Here's how the part is built. I have some questions about the finished solid (model axes, mm). Face numbers are marked on the shaded views. Round coordinates to 2 decimals unless told otherwise and drop trailing zeros. Loops run counter-clockwise (first coordinate to the right, second up) from the corner with the lowest first, then second, coordinate; pieces in that order, holes last. Notation, with made-up numbers: M 66.5,16 L 87.5,16 A16 cw 87.5,24 Z; hole C -15.75,-25 d9. An arc over 180 degrees is marked long. Use a Markdown table: item, result.
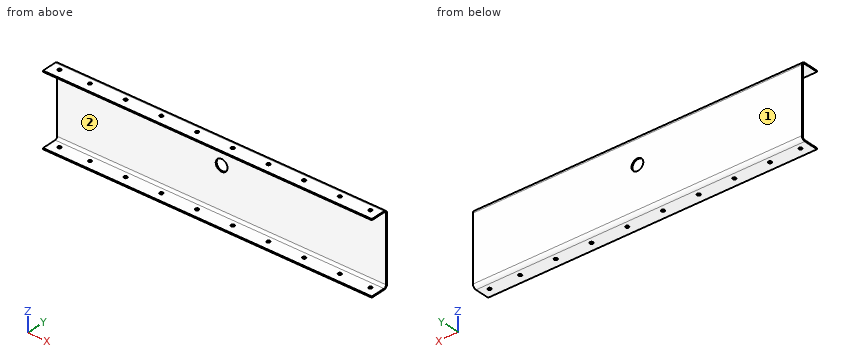
```python
from build123d import *

# Parameters (mm, degrees)
F1_DEPTH = 1400
F2_R     = 25
F3_DEPTH = 5
F4_R     = 7
F5_DEPTH = 305.001
F6_DEPTH = 305.001


with BuildPart() as f1:
    # F0 (on Right) → F1 (new body)
    with BuildSketch(Plane.YZ):
        with BuildLine():
            Line((0, 5), (0, 0))
            Line((0, 0), (62, 0))
            ThreePointArc((62, 0), (72.606602, 4.393398), (77, 15))
            Line((77, 15), (77, 290))
            ThreePointArc((77, 290), (72.606602, 300.606602), (62, 305))
            Line((62, 305), (0, 305))
            Line((0, 305), (0, 300))
            Line((0, 300), (62, 300))
            ThreePointArc((62, 300), (69.071068, 297.071068), (72, 290))
            Line((72, 290), (72, 15))
            ThreePointArc((72, 15), (69.071068, 7.928932), (62, 5))
            Line((62, 5), (0, 5))
        make_face()
    extrude(amount=F1_DEPTH)

    # F2 (on face) → F3 (cut, through all)
    with BuildSketch(Plane(origin=(0, 77, 0), x_dir=(-1, 0, 0), z_dir=(0, 1, 0))):
        with Locations((-700, 190)):
            Circle(F2_R)
    extrude(amount=-F3_DEPTH, mode=Mode.SUBTRACT)

    # F4 (on face) → F5 (cut, through all)
    with BuildSketch(Plane.XY.offset(305)):
        with BuildLine():
            ThreePointArc((783, 38), (771.050253, 42.949747), (776, 31))
            ThreePointArc((776, 31), (780.949747, 33.050253), (783, 38))
        make_face()
        with Locations((928, 38)):
            Circle(F4_R)
        with Locations((1080, 38)):
            Circle(F4_R)
        with Locations((1232, 38)):
            Circle(F4_R)
        with Locations((1362, 38)):
            Circle(F4_R)
    extrude(amount=-F5_DEPTH, mode=Mode.SUBTRACT)

    # F4 (on face) → F6 (cut, through all)
    with BuildSketch(Plane.XY.offset(305)):
        with BuildLine():
            ThreePointArc((776, 31), (780.949747, 33.050253), (783, 38))
            ThreePointArc((783, 38), (771.050253, 42.949747), (776, 31))
        make_face()
        with Locations((928, 38)):
            Circle(F4_R)
        with Locations((1080, 38)):
            Circle(F4_R)
        with Locations((1232, 38)):
            Circle(F4_R)
        with Locations((1362, 38)):
            Circle(F4_R)
        with Locations((624, 38)):
            Circle(F4_R)
        with Locations((472, 38)):
            Circle(F4_R)
        with Locations((320, 38)):
            Circle(F4_R)
        with Locations((168, 38)):
            Circle(F4_R)
        with Locations((38, 38)):
            Circle(F4_R)
    extrude(amount=-F6_DEPTH, mode=Mode.SUBTRACT)


solid = f1.part
```
Q1. Imagine slicing it at A-A, the plane z = 190. Please give me the cut outline in (x, y).
Return value:
| item | result |
|---|---|
| outline | M 0,72 L 675,72 L 675,77 L 0,77 Z; M 725,72 L 1400,72 L 1400,77 L 725,77 Z |
Q2. I need wall thicknesses on line 1 (Z direction, x = 1024, y = 7.5); line 2 (Y direction, x = 1232, z = 3.95); line 3 (Y direction, x = 349, z = 111). Which ranges of each line are inside material? Lowest first, please. Write a range as from..to.
Return value:
| item | result |
|---|---|
| line 1 | z = 0..5, 300..305 |
| line 2 | y = 0..31, 45..72.14 |
| line 3 | y = 72..77 |
Q3. Will these pins go through, and if not, where does the flat tip stop? P1, Ø11, axis at x = 320, y = 38, coming from the -Z side; P2, Ø1.5, axis at x = 777.5, z = 220.5, coming from the -Y side.
Return value:
| item | result |
|---|---|
| P1 | passes through |
| P2 | stops at y = 72 |
Q4. Imagine slicing it at B-B, the plane x = 1302. Please give me the cut outline in (y, z), then the cut area to 3 significant figures.
Return value:
| item | result |
|---|---|
| outline | M 0,0 L 62,0 A15 ccw 77,15 L 77,290 A15 ccw 62,305 L 0,305 L 0,300 L 62,300 A10 cw 72,290 L 72,15 A10 cw 62,5 L 0,5 Z |
| area | 2,190 mm^2 |
Q5. We'd pull the mould along Z, two halves only. Please class the marked faces 1 and 2: pulls with the +Z half, pulls with the -Z half, needs draft (parallel to the pull), parting line crosses it, or undercut.
Return value:
| item | result |
|---|---|
| face 1 | needs draft |
| face 2 | undercut |
Q6. Imagine slicing it at C-C, the plane z = 129.5. Please give me the cut outline in (x, y).
Return value:
| item | result |
|---|---|
| outline | M 0,72 L 1400,72 L 1400,77 L 0,77 Z |
